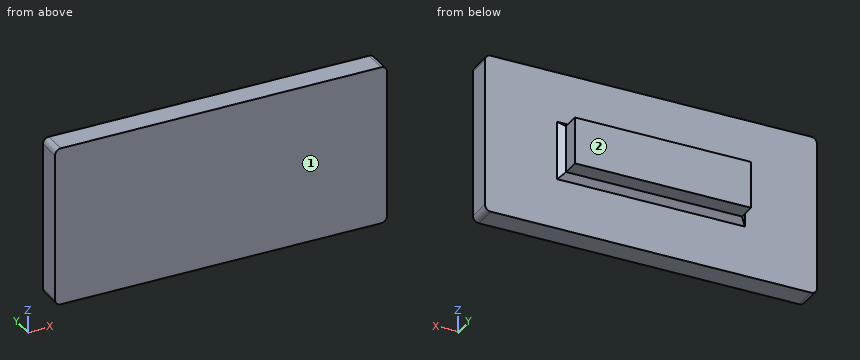
from build123d import *

# Parameters (mm, degrees)
SKETCH1_W           = 28.3
SKETCH1_H           = 13.6
BOSS_EXTRUDE1_DEPTH = 2
FILLET1_R           = 0.5
SKETCH2_W           = 15
SKETCH2_H           = 4
BOSS_EXTRUDE2_DEPTH = 2
CHAMFER1_SIZE       = 0.5


with BuildPart() as part:
    # Sketch1 → Boss-Extrude1 (new body)
    with BuildSketch(Plane(origin=(0, 0, 0), x_dir=(1, 0, 0), z_dir=(0, 1, 0))):
        Rectangle(SKETCH1_W, SKETCH1_H)
    extrude(amount=BOSS_EXTRUDE1_DEPTH)

    # Fillet1
    fillet1_edges = [part.edges().sort_by_distance(p)[0] for p in [
        (-14.15, 1, 6.8),
        (14.15, 1, 6.8),
        (14.15, 1, -6.8),
        (-14.15, 1, -6.8),
    ]]
    fillet(fillet1_edges, radius=FILLET1_R)

    # Sketch2 → Boss-Extrude2 (add)
    with BuildSketch(Plane(origin=(0, 2, 0), x_dir=(1, 0, 0), z_dir=(0, 1, 0))):
        Rectangle(SKETCH2_W, SKETCH2_H)
    extrude(amount=BOSS_EXTRUDE2_DEPTH)

    # Chamfer1
    chamfer1_edges = [part.edges().sort_by_distance(p)[0] for p in [
        (7.5, 2, 0),
        (0, 2, -2),
        (-7.5, 2, 0),
        (0, 2, 2),
    ]]
    chamfer(chamfer1_edges, length=CHAMFER1_SIZE)


solid = part.part
The listing builds one solid part. Answer for the finished solid, in the listing's coordinates (mm). Face numbers are marked on the shaded views. Give positions to 0.01 mm unless a question says otherwise; leave off trailing zeros. Loops run counter-clockwise (first coordinate to the right, second up) from the corner with the lowest first, then second, coordinate; pieces in that order, holes last. Notation, with made-up numbers: (-22, -6.75) - (27, -6.75) arc R17 ccw to (27, 6.25) - close; hole circle Ø3 at (72, 89.25). An arc over 180 degrees is marked (long way). Use one line per item in the form item = value.
1. Section C-C on y = 2.8 is taken. Give the vertices of the cut face in (x, z).
Calculated:
outline = (-7.5, -2) - (7.5, -2) - (7.5, 2) - (-7.5, 2) - close
2. Section A-A on z = -1 is taken. Give the vertices of the cut face in (x, y).
Calculated:
outline = (-14.15, 0) - (14.15, 0) - (14.15, 2) - (8, 2) - (7.5, 2.5) - (7.5, 4) - (-7.5, 4) - (-7.5, 2.5) - (-8, 2) - (-14.15, 2) - close
3. Find the intervals of material crossed by line 1 along Y through (x, z) = (-9.25, 0.5); line 2 along Z through (x, y) = (-1.5, 3.1); line 3 along X through (y, z) = (2.1, -0.75), in increasing order. Write a range as [from, to].
Calculated:
line_1 = [0, 2]
line_2 = [-2, 2]
line_3 = [-7.9, 7.9]
4. The mould has two halves that part along Y. Classify the marked faces 1 and 2: pulls with the +Y half, pulls with the -Y half, needs draft (parallel to the pull), parting line crosses it, or undercut.
Calculated:
face_1 = pulls with the -Y half
face_2 = pulls with the +Y half
5. Section D-D on z = 3 is taken. Give the vertices of the cut face in (x, y).
Calculated:
outline = (-14.15, 0) - (14.15, 0) - (14.15, 2) - (-14.15, 2) - close
6. Given pin 1 Ø0.8 at (x, y) = (2, 3) entering from +Z; pin 2 Ø0.8 at (y, z) = (3, -0.5) entering from -X; pin 3 Ø1.2 at (x, y) = (-3, 3.5) entering from -Z, each flat-ended and moving along its own axis, determine where each tip first touches the part or whether it passes through.
Calculated:
pin_1 = 2
pin_2 = -7.5
pin_3 = -2
7. Section B-B on x = -4.5 is taken. Give the vertices of the cut face in (y, z), then the cut area to 4 significant figures.
Calculated:
outline = (0, -6.8) - (2, -6.8) - (2, -2.5) - (2.5, -2) - (4, -2) - (4, 2) - (2.5, 2) - (2, 2.5) - (2, 6.8) - (0, 6.8) - close
area = 35.45 mm^2
